Autodesk Fusion 360 part; units mm, degrees
sketch "Sketch1" plane through (0, 0, 0) normal (0, 0, 1) x (1, 0, 0)
  circle A0 centre (0, 0) radius 16
  line L0 (0, 0) -> (19.5, 0) construction
  circle A1 centre (19.5, 0) radius 2
  line L1 (0, 0) -> (0, 16) construction
  circle A2 centre (-19.5, 0) radius 2
  line L2 (23.5, 5) -> (-23.5, 5)
  line L3 (-23.5, 5) -> (-23.5, -5)
  line L4 (-23.5, -5) -> (23.5, -5)
  line L5 (23.5, -5) -> (23.5, 5)
  line L6 (23.5, 5) -> (-23.5, -5) construction
  line L7 (-23.5, 5) -> (23.5, -5) construction
  circle A3 centre (0, 0) radius 19
  line L8 (-14.5, 5) -> (-24.5, 5)
  line L9 (-24.5, 5) -> (-24.5, -5)
  line L10 (-24.5, -5) -> (-14.5, -5)
  line L11 (-14.5, -5) -> (-14.5, 5)
  line L12 (-14.5, 5) -> (-24.5, -5) construction
  line L13 (-24.5, 5) -> (-14.5, -5) construction
  line L14 (24.5, 5) -> (24.5, -5)
  line L15 (24.5, -5) -> (14.5, -5)
  line L16 (14.5, -5) -> (14.5, 5)
  line L17 (14.5, 5) -> (24.5, 5)
  line L18 (-14.5, -5) -> (-14.5, -6.7639)
  line L19 (-14.5, 5) -> (-14.5, 6.7639)
  line L20 (14.5, 5) -> (14.5, 6.7639)
  line L21 (14.5, -5) -> (14.5, -6.7639)
  point P0 (-19.5, 0)
  dimension "d1" = 32
  dimension "d2" = 19.5
  dimension "d3" = 4
  dimension "d4" = 3
  dimension "d5" = 4
  dimension "d6" = 10
  dimension "d11" = 5
extrude "Extrude1" add sketch "Sketch1" along normal blind 3.2 contours A0 L2 A3 L8 L17 | A0 L2 L17 L20 | A0 L2 L8 L19 | A0 A1 L2 L4 A3 L15 L17 | A0 L2 L4 L15 L16 L17 | A0 L2 L4 L8 L10 L11 | A0 A2 L2 L4 A3 L8 L10 | A1 L2 L4 L5 A3 L15 L17 | A0 L4 L15 L21 | A0 L4 L10 L18 | A0 L4 A3 L10 L15 | A2 L2 L3 L4 A3 L8 L10
fillet "Fillet1" radius 2 4 edges at (-23.5, -5, 1.6) (-23.5, 5, 1.6) (23.5, -5, 1.6) (23.5, 5, 1.6)
equation "d2 = ( 39 / 2 ) * 1 mm"
Build history of the part. All positions in model axes, mm. A direction names the side the tool comes from. Coordinates: 2 decimals unless noted, no trailing zeros. Write each loop counter-clockwise with the first axis right and the second up, starting at its lowest first coordinate (ties: lowest second). Pieces come first, ordered by that corner, then holes.
1. Drill centre lines: probe 1 along X at (y, z) = (0, 2.35); probe 2 along Y at (x, z) = (-0.5, 2.7); probe 3 along Y at (x, z) = (19.5, 1.5). Where is each one in solid material? Low to high.
Answer block:
probe 1: x = -23.5 to -21.5, -17.5 to -14.5, 14.5 to 17.5, 21.5 to 23.5
probe 2: y = -18.99 to -15.99, 15.99 to 18.99
probe 3: y = -5 to -2, 2 to 5
2. 3-axis set-ups, long thin cutter, end or side, ignore diameter. For faces 1 (the flat face through (14.5, 0, 2)), 2 (the flat face through (-23.5, 0, 2)), 3 (the flat face through (20, -5, 2)), 4 (the flat face through (-16, -1, 0)), 5 (the flat face through (-20, 5, 2)): which of +Z, -Z, +X, -X, +Y, -Y reach the whole face in a straight line?
Answer block:
face 1: +Z, -Z
face 2: +Z, -Z, -X, +Y, -Y
face 3: +Z, -Z, +X, -Y
face 4: -Z, +X, -X, +Y, -Y
face 5: +Z, -Z, -X, +Y
3. Band-saw the part on A-A, the plane y = 0. Give the cut face in (x, z), and give its area (3 significant figures).
Answer block:
outline: (-23.5, 0) - (-21.5, 0) - (-21.5, 3.2) - (-23.5, 3.2) - close; (-17.5, 0) - (-14.5, 0) - (-14.5, 3.2) - (-17.5, 3.2) - close; (14.5, 0) - (17.5, 0) - (17.5, 3.2) - (14.5, 3.2) - close; (21.5, 0) - (23.5, 0) - (23.5, 3.2) - (21.5, 3.2) - close
area: 32.0 mm2
4. Band-saw the part on D-D, the plane y = -9. Give the cut face in (x, z), and give its area (3 significant figures).
Answer block:
outline: (-16.73, 0) - (-13.23, 0) - (-13.23, 3.2) - (-16.73, 3.2) - close; (13.23, 0) - (16.73, 0) - (16.73, 3.2) - (13.23, 3.2) - close
area: 22.4 mm2
5. Band-saw the part on C-C, the plane z = 2.05. Give the cut face in (x, y).
Answer block:
outline: (-23.5, -3) arc R2 ccw to (-21.5, -5) - (-18.33, -5) arc R19 ccw to (18.33, -5) - (21.5, -5) arc R2 ccw to (23.5, -3) - (23.5, 3) arc R2 ccw to (21.5, 5) - (18.33, 5) arc R19 ccw to (-18.33, 5) - (-21.5, 5) arc R2 ccw to (-23.5, 3) - close; hole circle Ø4 at (-19.5, 0); hole (-14.5, -6.76) arc R16 ccw to (14.5, -6.76) - (14.5, 6.76) arc R16 ccw to (-14.5, 6.76) - close; hole circle Ø4 at (19.5, 0)
6. Drop flat-ended pins along their axis: pin 1 (3.5 mm diameter, centred on x = -19.5, y = 0, fed in from -Z); pin 2 (1 mm diameter, centred on x = 20.5, z = 2, fed in from +Y); pin 3 (1 mm diameter, centred on x = -19.5, z = 1.5, fed in from -Y). Give the stop position or say it passes through.
Answer block:
pin 1: passes through
pin 2: stops at y = 5
pin 3: stops at y = -5
7. Band-saw the part on B-B, the plane x = 19.5. Give the cut face in (y, z), and give its area (3 significant figures).
Answer block:
outline: (-5, 0) - (-2, 0) - (-2, 3.2) - (-5, 3.2) - close; (2, 0) - (5, 0) - (5, 3.2) - (2, 3.2) - close
area: 19.2 mm2
8. Pull direction X, two halves, no side cores. Call faces 6 (the cylindrical face through (22.93, 4.4, 1.62)), 7 (the flat face through (-20, -5, 2)), 8 (the cylindrical face through (0, -16, 2)), 9 (the cylindrical face through (-22.9, 4.43, 1.62)): released by +X, released by -X, zero draft, split by the parting line, or undercut.
Answer block:
face 6: released by +X
face 7: zero draft
face 8: undercut
face 9: released by -X
